Verification items for this drawing (mm, ordinates from the low corner). A direction names the side the tool comes from. Give positions to 0.01 mm unless a question says otherwise; leave off trailing zeros. Loops run counter-clockwise (first coordinate to the right, second up) from the corner with the lowest first, then second, coordinate; pieces in that order, holes last. Notation, with made-up numbers: (46.5, 40) -> (50.5, 40) arc R13 ccw to (50.5, 45) -> close; hole circle Ø6 at (-30, 51). An arc over 180 degrees is marked (long way). Write each question's results on one line, items separated by ' | '. Start each with the question number.
Item 1: Cross-section at D-D on z = 18. Enter the section's corners in (x, y).
Item 2: Cross-section at B-B on x = 49. Enter the section's corners in (y, z), then the cut area to 3 significant figures.
Item 3: Cross-section at A-A on z = 15. Enter the section's corners in (x, y), then the cut area to 3 significant figures.
Item 4: Scan lines: line 1 along X through (y, z) = (3.7, 15); line 2 along X through (y, z) = (11.5, 28.25); line 3 along Z through (x, y) = (5, 3.1). Record each from-to range of solid material in increasing order.
Item 5: Access from +Z, -Z, +X, -X, +Y, -Y to the whole of each face (thin tool, end or side, straight path). Record for the marked faces 5, 6 and 7.
Item 6: Gauge pin test, flat ends, axial feed: pin 1 Ø5 at (y, z) = (9, 23) entering from -X; pin 2 Ø5 at (x, z) = (49.5, 20.5) entering from +Y; pin 3 Ø10 at (x, z) = (8.5, 25) entering from -Y; pin 4 Ø3.5 at (y, z) = (8, 14) entering from +X. Record the tip position at first contact, or that the pin passes through.
Item 7: Cross-section at C-C on y = 13. Enter the section's corners in (x, z), then the cut area to 3 significant figures.
Item 8: Mould release check, pull along Z, two halves, no side actions. Record for the marked faces 1, 2, 3 and 4: pulls with the +Z half, pulls with the -Z half, needs draft (parallel to the pull), parting line crosses it, or undercut.
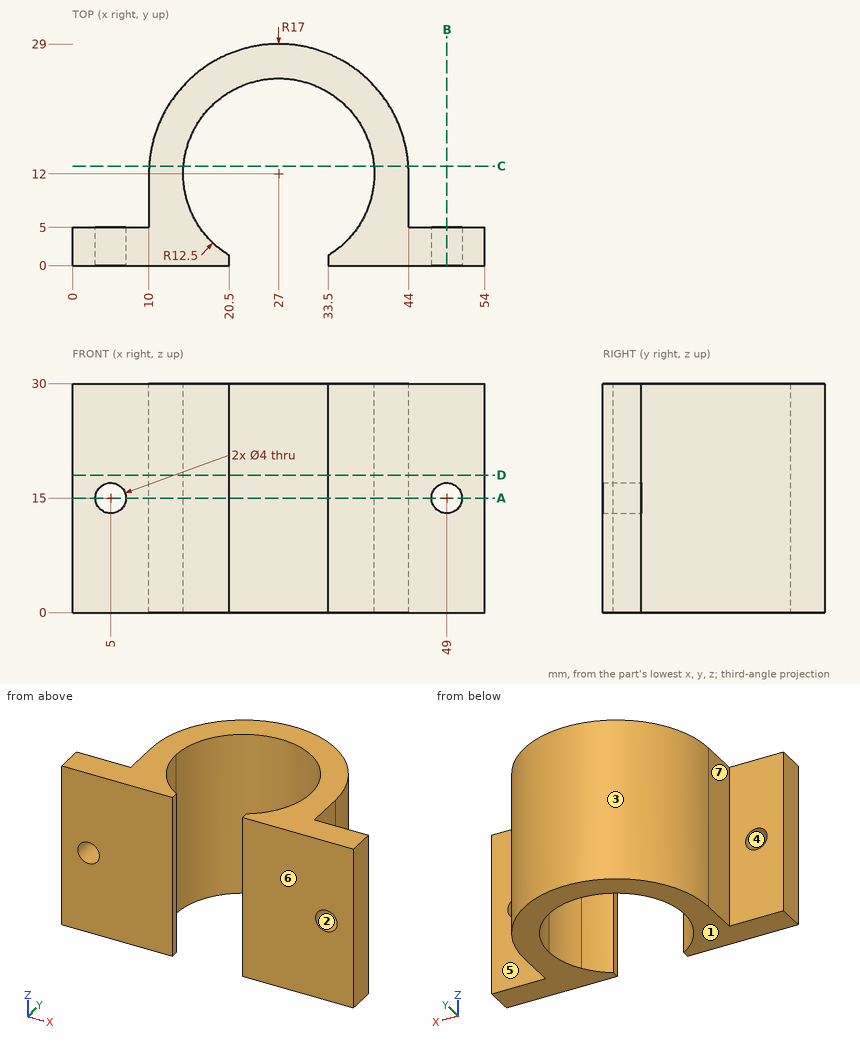
Answer sheet:
1) outline: (0, 0) -> (20.5, 0) -> (20.5, 1.32) arc R12.5 cw (long way) to (33.5, 1.32) -> (33.5, 0) -> (54, 0) -> (54, 5) -> (44, 5) -> (44, 12) arc R17 ccw to (10, 12) -> (10, 5) -> (0, 5) -> close
2) outline: (0, 0) -> (5, 0) -> (5, 13) -> (0, 13) -> close; (0, 17) -> (5, 17) -> (5, 30) -> (0, 30) -> close | area: 130 mm²
3) outline: (0, 0) -> (3, 0) -> (3, 5) -> (0, 5) -> close; (7, 0) -> (20.5, 0) -> (20.5, 1.32) arc R12.5 cw (long way) to (33.5, 1.32) -> (33.5, 0) -> (47, 0) -> (47, 5) -> (44, 5) -> (44, 12) arc R17 ccw to (10, 12) -> (10, 5) -> (7, 5) -> close; (51, 0) -> (54, 0) -> (54, 5) -> (51, 5) -> close | area: 430 mm²
4) line 1: x = 0 to 3, 7 to 17.65, 36.35 to 47, 51 to 54 | line 2: x = 10 to 14.51, 39.49 to 44 | line 3: z = 0 to 13, 17 to 30
5) face 5: +Z, -Z, +X, +Y | face 6: +Z, -Z, +X, -X, -Y | face 7: +Z, -Z, -X, +Y
6) pin 1: stops at x = 10 | pin 2: stops at y = 5 | pin 3: stops at y = 0 | pin 4: stops at x = 44
7) outline: (10.03, 0) -> (14.54, 0) -> (14.54, 30) -> (10.03, 30) -> close; (39.46, 0) -> (43.97, 0) -> (43.97, 30) -> (39.46, 30) -> close | area: 271 mm²
8) face 1: pulls with the -Z half | face 2: undercut | face 3: needs draft | face 4: undercut
